```python
from build123d import *

# Parameters (mm, degrees)
EXTRUDE_1_DEPTH     = 4.35
CUT_EXTRUDE_START   = -2.195068
SKETCH_2_W          = 7.909800434
SKETCH_2_H          = 2.721108573
SKETCH_2_W_2        = 2.301330542
SKETCH_2_H_2        = 4.187137181
SKETCH_2_W_3        = 4.35
CUT_EXTRUDE_1_DEPTH = 13.336862915
FILLET_1_R          = 0.5
EXTRUDE_START       = 4.707534
SKETCH_3_R          = 0.25
EXTRUDE_2_DEPTH     = 7.3


with BuildPart() as part:
    # Эскиз1 → Бобышка-Вытянуть1 (new, symmetric)
    with BuildSketch(Plane(origin=(0, 0, 0), x_dir=(0, 0, -1), z_dir=(1, 0, 0))):
        with BuildLine():
            Line((-2.195067928, 0), (-2.195067928, 4.207534134))
            ThreePointArc((-2.195067928, 4.207534134), (-2.048621319, 4.561087525), (-1.695067928, 4.707534134))
            Line((-1.695067928, 4.707534134), (-1.048425102, 4.707534134))
            Line((-1.048425102, 4.707534134), (-1.048425102, 8.894671315))
            Line((-1.048425102, 8.894671315), (1.048425102, 8.894671315))
            Line((1.048425102, 8.894671315), (1.048425102, 4.707534134))
            Line((1.048425102, 4.707534134), (1.695067928, 4.707534134))
            ThreePointArc((1.695067928, 4.707534134), (2.048621319, 4.561087525), (2.195067928, 4.207534134))
            Line((2.195067928, 4.207534134), (2.195067928, 0))
            Line((2.195067928, 0), (1.245504338, 0))
            ThreePointArc((1.245504338, 0), (0.813528527, 0.431975811), (0.381552716, 0))
            add(Edge.make_bspline(
                [(0.381552716, 0), (0.533291167, -0.533550096), (0.61904307, -1.408984288), (0.53277478, -2.660476036), (0, -2.721108573)],
                knots=[0, 0, 0, 0, 0.537169864, 1, 1, 1, 1], degree=3))
            add(Edge.make_bspline(
                [(-0.381552716, 0), (-0.533291167, -0.533550096), (-0.61904307, -1.408984288), (-0.53277478, -2.660476036), (0, -2.721108573)],
                knots=[0, 0, 0, 0, 0.537169864, 1, 1, 1, 1], degree=3))
            ThreePointArc((-0.381552716, 0), (-0.813528527, 0.431975811), (-1.245504338, 0))
            Line((-1.245504338, 0), (-2.195067928, 0))
        make_face()
    extrude(amount=EXTRUDE_1_DEPTH, both=True)

    # Эскиз2 → Вырез-Вытянуть1 (cut, through all)
    with BuildSketch(Plane.XY.offset(CUT_EXTRUDE_START)):
        with Locations((0, -1.360554286)):
            Rectangle(SKETCH_2_W, SKETCH_2_H)
        with Locations((-3.199334729, 6.801102724)):
            Rectangle(SKETCH_2_W_2, SKETCH_2_H_2)
        with Locations((2.175, 6.801102724)):
            Rectangle(SKETCH_2_W_3, SKETCH_2_H_2)
    extrude(amount=CUT_EXTRUDE_1_DEPTH, mode=Mode.SUBTRACT)

    # Скругление1
    fillet_1_edges = [part.edges().sort_by_distance(p)[0] for p in [
        (-4.35, 2.103767067, 2.195067928),
        (-4.35, 4.561087525, 2.048621319),
        (-4.35, 4.707534134, 0),
        (-4.35, 4.561087525, -2.048621319),
        (-4.35, 2.103767067, -2.195067928),
        (4.35, 2.103767067, -2.195067928),
        (4.35, 4.561087525, -2.048621319),
        (4.35, 4.707534134, 0),
        (4.35, 4.561087525, 2.048621319),
        (4.35, 2.103767067, 2.195067928),
    ]]
    fillet(fillet_1_edges, radius=FILLET_1_R)

    # Эскиз3 → Бобышка-Вытянуть2 (add)
    with BuildSketch(Plane(origin=(0, 0, 0), x_dir=(1, 0, 0), z_dir=(0, 1, 0)).offset(EXTRUDE_START)):
        with Locations(Location((0, 0, 0), (0, 0, 90))):
            Circle(SKETCH_3_R)
        with Locations(Location((-2, 0, 0), (0, 0, 90))):
            Circle(SKETCH_3_R)
        with Locations(Location((2, 0, 0), (0, 0, 90))):
            Circle(SKETCH_3_R)
    extrude(amount=-EXTRUDE_2_DEPTH)


solid = part.part
```
Build history of the part. All positions in model axes, mm. A direction names the side the tool comes from. Give positions to 0.01 mm unless a question says otherwise; leave off trailing zeros. Loops run counter-clockwise (first coordinate to the right, second up) from the corner with the lowest first, then second, coordinate; pieces in that order, holes last.
1) Two-plate mould, pull along Z, no slides. Class faces 4 (the face through (0, 7, 0)), 5 (the face through (0.06, 0.43, 0.8)), 6 (the face through (-1, 7, -1.048)): released by +Z, released by -Z, zero draft, split by the parting line, or undercut.
Values follow:
face 4: zero draft
face 5: undercut
face 6: released by -Z
2) Band-saw the part on C-C on y = 5.75. List the corners of the cut face in (x, z).
Values follow:
outline: (-2.05, -1.05) - (0, -1.05) - (0, 1.05) - (-2.05, 1.05) - close
3) Band-saw the part on B-B on z = -0.8. List the corners of the cut face in (x, y).
Values follow:
outline: (-4.35, 0.43) - (4.35, 0.43) - (4.35, 4.21) arc R0.5 ccw to (3.85, 4.71) - (0, 4.71) - (0, 8.89) - (-2.05, 8.89) - (-2.05, 4.71) - (-3.85, 4.71) arc R0.5 ccw to (-4.35, 4.21) - close
4) Probe line 1 along Z through (x, y) = (-2, -2); line 2 along X through (y, z) = (4.75, 0.4); line 3 along Y through (x, z) = (3, -1.45). List the from-to ranges inside material, lowest first.
Values follow:
line 1: z = -0.25 to 0.25
line 2: x = -2.05 to 0
line 3: y = 0 to 4.71
5) Band-saw the part on A-A on x = 2. List the corners of the cut face in (y, z).
Values follow:
outline: (-2.59, -0.25) - (0, -0.25) - (0, -0.38) arc R0.43 cw to (0, -1.25) - (0, -2.2) - (4.21, -2.2) arc R0.5 ccw to (4.71, -1.7) - (4.71, 1.7) arc R0.5 ccw to (4.21, 2.2) - (0, 2.2) - (0, 1.25) arc R0.43 cw to (0, 0.38) - (0, 0.25) - (-2.59, 0.25) - close
6) Drop flat-ended pins along their axis: P1, Ø2.5, axis at y = 7.5, z = 0, coming from the -X side; P2, Ø2.5, axis at x = -1, y = 6, coming from the -Z side; P3, Ø1, axis at y = 7, z = 0, coming from the +X side. Give the stop position or say it passes through.
Values follow:
P1: stops at x = -2.05
P2: stops at z = -1.05
P3: stops at x = 0
7) 3-axis set-ups, long thin cutter, end or side, ignore diameter. For faces 1 (the face through (-3.955, -1, 0)), 2 (the face through (-2.049, 7, 0)), 3 (the face through (-1, 7, 1.048)): which of +Z, -Z, +X, -X, +Y, -Y reach the whole face in a straight line?
Values follow:
face 1: +Z, -Z, -Y
face 2: +Z, -Z, -X, +Y
face 3: +Z, +X, -X, +Y
